Read the model definition and answer for the solid it produces. Units are mm, in the model's axes. A direction names the side the tool comes from. Round coordinates to 2 decimals unless told otherwise and drop trailing zeros. Order: outer loops, then holes, each group sorted by start corner. A loop starts at its lowest first (then second) coordinate and runs counter-clockwise, first axis right, second up. Notation, with made-up numbers: M 42.25,70.25 L 76.25,70.25 A27 ccw 76.25,88.25 Z; hole C -12.75,84.25 d11. An arc over 180 degrees is marked long. Answer as CSV lines item,"result".
```python
from build123d import *

# Parameters (mm, degrees)
F1_DEPTH = 228.6
F0_W     = 14.8112885654
F0_H     = 40.948856622
F0_W_2   = 2.9041729867
F0_W_3   = 24.6854852885
F0_W_4   = 4.3562594801
F0_W_5   = 24.3950609583
F0_W_6   = 6.6796054598
F0_W_7   = 55.7601368055
F2_DEPTH = 2.54


with BuildPart() as f1:
    # F0 (on Top) → F1 (new body)
    with BuildSketch(Plane.XY):
        Polygon((65.9247487783, 20.474428311), (74.3468627334, 20.474428311), (74.3468627334, 24.8306896538), (-74.3468627334, 24.8306896538), (-74.3468627334, 20.474428311), (-67.667260766, 20.474428311), (-52.8559722006, 20.474428311), (-49.9517992139, 20.474428311), (-25.2663139254, 20.474428311), (-20.9100544453, 20.474428311), (3.4850065131, 20.474428311), (10.1646119729, 20.474428311), align=None)
    extrude(amount=F1_DEPTH)

    # F0 (on Top) → F2 (join)
    with BuildSketch(Plane.XY):
        Polygon((65.9247487783, -24.8306896538), (74.3468627334, -24.8306896538), (74.3468627334, 20.474428311), (65.9247487783, 20.474428311), (65.9247487783, -20.474428311), align=None)
        Polygon((-67.667260766, -24.8306896538), (65.9247487783, -24.8306896538), (65.9247487783, -20.474428311), (10.1646119729, -20.474428311), (3.4850065131, -20.474428311), (-20.9100544453, -20.474428311), (-25.2663139254, -20.474428311), (-49.9517992139, -20.474428311), (-52.8559722006, -20.474428311), (-67.667260766, -20.474428311), align=None)
        Polygon((65.9247487783, 20.474428311), (74.3468627334, 20.474428311), (74.3468627334, 24.8306896538), (-74.3468627334, 24.8306896538), (-74.3468627334, 20.474428311), (-67.667260766, 20.474428311), (-52.8559722006, 20.474428311), (-49.9517992139, 20.474428311), (-25.2663139254, 20.474428311), (-20.9100544453, 20.474428311), (3.4850065131, 20.474428311), (10.1646119729, 20.474428311), align=None)
        Polygon((-74.3468627334, -24.8306896538), (-67.667260766, -24.8306896538), (-67.667260766, -20.474428311), (-67.667260766, 20.474428311), (-74.3468627334, 20.474428311), align=None)
        with Locations((-60.2616164833, 0)):
            Rectangle(F0_W, F0_H)
        with Locations((-51.4038857073, 0)):
            Rectangle(F0_W_2, F0_H)
        with Locations((-37.6090565696, 0)):
            Rectangle(F0_W_3, F0_H)
        with Locations((-23.0881841853, 0)):
            Rectangle(F0_W_4, F0_H)
        with Locations((-8.7125239661, 0)):
            Rectangle(F0_W_5, F0_H)
        with Locations((6.824809243, 0)):
            Rectangle(F0_W_6, F0_H)
        with Locations((38.0446803756, 0)):
            Rectangle(F0_W_7, F0_H)
    extrude(amount=F2_DEPTH)


solid = f1.part
```
Item 1: A cutting plane is placed at A-A, the plane x = 2. Determine the outline of the cut face in (y, z).
Ans:
outline,"M -24.83,0 L 24.83,0 L 24.83,228.6 L 20.47,228.6 L 20.47,2.54 L -24.83,2.54 Z"
Item 2: Flat-ended cylindrical pins translate along their axes: pin 1 (22.5 mm diameter, centred on x = -27, y = -3.5, fed in from +Z); pin 2 (3 mm diameter, centred on x = 16.5, z = 32.5, fed in from -Y). Find the tip coordinate at first contact, or state that the pin passes through.
Ans:
pin 1,"z = 2.54"
pin 2,"y = 20.47"
Item 3: Find the intervals of material crossed by probe 1 along Y at (x, z) = (-53, 211); probe 2 along Z at (x, y) = (-24, -5), in increasing order. Write a range as [from, to].
Ans:
probe 1,"[20.47, 24.83]"
probe 2,"[0, 2.54]"
Item 4: A cutting plane is placed at B-B, the plane y = 14.5. Determine the outline of the cut face in (x, z), and give its area (3 significant figures).
Ans:
outline,"M -74.35,0 L 74.35,0 L 74.35,2.54 L -74.35,2.54 Z"
area,"378 mm2"
Item 5: A cutting plane is placed at C-C, the plane z = 27. Determine the outline of the cut face in (x, y).
Ans:
outline,"M -74.35,20.47 L 74.35,20.47 L 74.35,24.83 L -74.35,24.83 Z"
Item 6: A tool of negligible diameter and unlimited length cuts with its end or side. For faces 1 (the face through (-1, 20.474, 114)), 2 (the face through (74.347, 22, 114)), from which of +Z, -Z, +X, -X, +Y, -Y can it reach the whole face along a straight path? Write none if from no direction.
Ans:
face 1,"+Z, +X, -X, -Y"
face 2,"+Z, -Z, +X, +Y, -Y"
